Source: CAD feature listing. Evaluate the final solid. Frame: model axes, mm. Face numbers are marked on the shaded views. A direction names the side the tool comes from. Coordinates: 2 decimals unless noted, no trailing zeros. Order: outer loops, then holes, each group sorted by start corner. A loop starts at its lowest first (then second) coordinate and runs counter-clockwise, first axis right, second up. Notation, with made-up numbers: (58.25, 10.5) -> (84.25, 10.5) arc R12 cw to (84.25, 20.5) -> close; hole circle Ø11 at (16, -20). An arc over 180 degrees is marked (long way). Write item = value, one per line. Start each with the question number.
Item 1: Ray query, line 1 along X through (y, z) = (-1, -14); line 2 along Z through (x, y) = (36.5, 43); line 3 along Z through (x, y) = (11.5, 23.5). Return the intervals inside material, ascending. Write a range as [from, to].
Item 2: Section query A-A (z = 11.5). Output: boundary loops of the cut face in (x, y).
Item 3: Section query B-B (x = 25). Count the separate pieces of the cut face and the enclosed holes in it, then the cut area to 3 significant figures.
Item 4: Contact query for flat-ended pins moving along their axis: pin 1 (8 mm diameter, centred on x = 35.5, z = 17, fed in from -Y); pin 2 (3 mm diameter, centred on x = 19, z = -9.5, fed in from +Y); pin 3 (0.8 mm diameter, centred on x = 25.5, y = 19, fed in from -Z); pin 4 (3 mm diameter, centred on x = 25, z = -14, fed in from +Y). Output: stop coordinate, or through.
Item 5: Mould query, pull axis Z, two halves, no side actions, for the marked faces 4, 5 and 6. Classes: released by +Z, released by -Z, zero draft, split by the parting line, or undercut.
Item 6: Set-up query: the marked faces 1, 2 and 3. Return all of +Z, -Z, +X, -X, +Y, -Y with unobstructed straight access to the full face (end or side cutting, diameter ignored); none if empty.
Item 7: Section query D-D (z = -14). Output: boundary loops of the cut face in (x, y).
Item 8: Section query C-C (y = 42). Output: boundary loops of the cut face in (x, z).
```python
from build123d import *

# Parameters (mm, degrees)
EXTRUDE_1_DEPTH     = 6
SKETCH_2_W          = 50.01074492
SKETCH_2_H          = 5
EXTRUDE_2_DEPTH     = 30
SKETCH_4_R          = 1.75
CUT_EXTRUDE_1_DEPTH = 30
EXTRUDE_START       = 1.5
SKETCH_6_W          = 10
SKETCH_6_H          = 6
SKETCH_6_R          = 1.75
EXTRUDE_4_DEPTH     = 1.5
EXTRUDE_6_DEPTH     = 50
CUT_EXTRUDE_2_REACH = 105.013
SKETCH_15_W         = 1.024057277
SKETCH_15_H         = 0.768849672
EXTRUDE_10_DEPTH    = 20
EXTRUDE_11_DEPTH    = 6
SKETCH_17_W         = 10
SKETCH_17_H         = 6
SKETCH_17_R         = 1.75
EXTRUDE_12_DEPTH    = 1.5
CUT_EXTRUDE_START   = -100
SKETCH_18_R         = 1.75
CUT_EXTRUDE_3_DEPTH = 100


with BuildPart() as part:
    # Эскиз1 → Бобышка-Вытянуть1 (new body)
    with BuildSketch(Plane.XY):
        Polygon((0, 0), (8.5, 0), (11.5, 0), (38.5, 0), (41.5, 0), (50, 0), (50, 10), (50, 30), (30, 30), (20, 30), (0, 30), (0, 10), align=None)
        with BuildLine():
            Line((28, 22.5), (28, 7.5))
            ThreePointArc((28, 7.5), (25, 4.5), (22, 7.5))
            Line((22, 7.5), (22, 22.5))
            ThreePointArc((22, 22.5), (25, 25.5), (28, 22.5))
        make_face(mode=Mode.SUBTRACT)
    extrude(amount=EXTRUDE_1_DEPTH)

    # Эскиз2 → Бобышка-Вытянуть2 (add)
    with BuildSketch(Plane.XY.offset(6)):
        with Locations((25.00537246, -2.5)):
            Rectangle(SKETCH_2_W, SKETCH_2_H)
    extrude(amount=-EXTRUDE_2_DEPTH)

    # Эскиз4 → Вырез-Вытянуть1 (cut)
    with BuildSketch(Plane(origin=(0, 0, 0), x_dir=(1, 0, 0), z_dir=(0, 1, 0))):
        with Locations(Location((25, 14, 0), (0, 0, 270))):
            Circle(SKETCH_4_R)
    extrude(amount=-CUT_EXTRUDE_1_DEPTH, mode=Mode.SUBTRACT)

    # Эскиз6 → Бобышка-Вытянуть4 (add)
    with BuildSketch(Plane(origin=(0, 0, 0), x_dir=(1, 0, 0), z_dir=(0, 1, 0)).offset(EXTRUDE_START)):
        with Locations((25, 14)):
            Rectangle(SKETCH_6_W, SKETCH_6_H)
        with Locations(Location((25, 14, 0), (0, 0, 270))):
            Circle(SKETCH_6_R, mode=Mode.SUBTRACT)
    extrude(amount=-EXTRUDE_4_DEPTH)

    # Эскиз7 → Бобышка-Вытянуть6 (add)
    with BuildSketch(Plane.ZY):
        Polygon((58, -5), (58, 68.895321777), (0, 68.895321777), (0, 62.524087888), (0, -5), (6, -5), (6, 62.524087888), (52, 62.524087888), (52, -5), align=None)
    extrude(amount=-EXTRUDE_6_DEPTH)

    # Вырез-Вытянуть2: up to this face of the body (flat: up to its plane)
    cut_extrude_2_end = Plane(part.part.faces().sort_by_distance((25, 31.947660889, 58))[0])
    # Эскиз8 → Вырез-Вытянуть2 (cut, up to the picked face)
    with BuildSketch(Plane(origin=(0, 0, 0), x_dir=(-1, 0, 0), z_dir=(0, 0, -1)), mode=Mode.PRIVATE) as cut_extrude_2_sk1:
        with BuildLine():
            Line((-26.5, 112.5), (-23.5, 112.5))
            Line((-23.5, 112.5), (-23.5, 7.5))
            ThreePointArc((-23.5, 7.5), (-25, 5.175598625), (-26.5, 7.5))
            Line((-26.5, 7.5), (-26.5, 112.5))
        make_face()
    cut_extrude_2_tool1 = split(extrude(cut_extrude_2_sk1.sketch, amount=-CUT_EXTRUDE_2_REACH, mode=Mode.PRIVATE), bisect_by=cut_extrude_2_end, keep=Keep.BOTH, mode=Mode.PRIVATE)
    add(cut_extrude_2_tool1.solids().sort_by(Axis((25, 58.930041, 0), (0, 0, 1)))[0], mode=Mode.SUBTRACT)

    # Эскиз15 → Бобышка-Вытянуть10 (add)
    with BuildSketch(Plane(origin=(0, 0, 0), x_dir=(1, 0, 0), z_dir=(0, 1, 0))):
        with Locations((49.487971362, 0.384424836)):
            Rectangle(SKETCH_15_W, SKETCH_15_H)
    extrude(amount=EXTRUDE_10_DEPTH)

    # Эскиз16 → Бобышка-Вытянуть11 (add)
    with BuildSketch(Plane(origin=(0, 20, 0), x_dir=(1, 0, 0), z_dir=(0, 1, 0))):
        Polygon((50, 0), (28.5, 0), (28.5, 4), (21.5, 4), (21.5, 0), (0, 0), (0, 24), (50, 24), align=None)
    extrude(amount=EXTRUDE_11_DEPTH)

    # Эскиз17 → Бобышка-Вытянуть12 (add)
    with BuildSketch(Plane.XZ.offset(-20)):
        with Locations((25, -14)):
            Rectangle(SKETCH_17_W, SKETCH_17_H)
        with Locations(Location((25, -14, 0), (0, 0, 90))):
            Circle(SKETCH_17_R, mode=Mode.SUBTRACT)
    extrude(amount=EXTRUDE_12_DEPTH)

    # Эскиз18 → Вырез-Вытянуть3 (cut)
    with BuildSketch(Plane.XZ.offset(-18.5).offset(CUT_EXTRUDE_START)):
        with Locations(Location((25, -14, 0), (0, 0, 90))):
            Circle(SKETCH_18_R)
    extrude(amount=CUT_EXTRUDE_3_DEPTH, mode=Mode.SUBTRACT)


solid = part.part
```
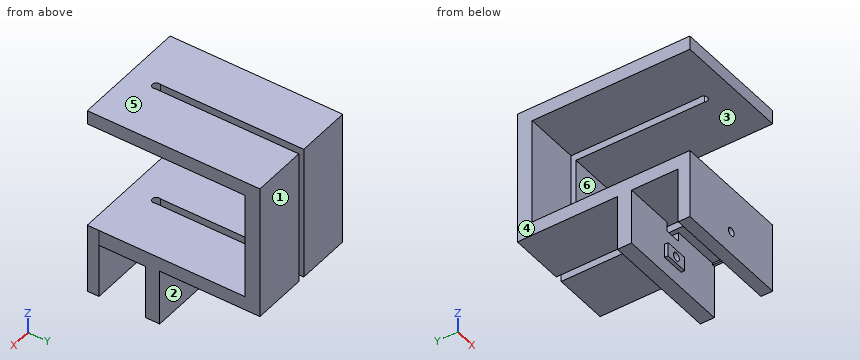
Computed:
q1.line_1 = [0, 23.25], [26.75, 50.01]
q1.line_2 = [0, 6], [52, 58]
q1.line_3 = [-24, 6], [52, 58]
q2.outline = (0, 62.52) -> (23.5, 62.52) -> (23.5, 68.9) -> (0, 68.9) -> close; (26.5, 62.52) -> (50, 62.52) -> (50, 68.9) -> (26.5, 68.9) -> close
q3.separate_pieces = 5
q3.enclosed_holes = 0
q3.area = 331 mm^2
q4.pin_1 = 62.52
q4.pin_2 = 26
q4.pin_3 = -17
q4.pin_4 = through
q5.face_4 = zero draft
q5.face_5 = released by +Z
q5.face_6 = undercut
q6.face_1 = +Z, -Z, +X, -X, +Y
q6.face_2 = -Z, +X, -X, +Y
q6.face_3 = +X, -X, -Y
q7.outline = (0, -5) -> (23.25, -5) -> (23.25, 1.5) -> (20, 1.5) -> (20, 0) -> (0, 0) -> close; (0, 20) -> (20, 20) -> (20, 18.5) -> (23.25, 18.5) -> (23.25, 26) -> (0, 26) -> close; (26.75, -5) -> (50.01, -5) -> (50.01, 0) -> (30, 0) -> (30, 1.5) -> (26.75, 1.5) -> close; (26.75, 18.5) -> (30, 18.5) -> (30, 20) -> (50, 20) -> (50, 26) -> (26.75, 26) -> close
q8.outline = (0, 0) -> (23.5, 0) -> (23.5, 6) -> (0, 6) -> close; (0, 52) -> (23.5, 52) -> (23.5, 58) -> (0, 58) -> close; (26.5, 0) -> (50, 0) -> (50, 6) -> (26.5, 6) -> close; (26.5, 52) -> (50, 52) -> (50, 58) -> (26.5, 58) -> close
